Autodesk Inventor part; units mm, degrees
ref_plane "YZ Plane" through (0, 0, 0) normal (1, 0, 0) x (0, 1, 0)
ref_plane "XZ Plane" through (0, 0, 0) normal (0, 1, 0) x (-1, 0, 0)
ref_plane "XY Plane" through (0, 0, 0) normal (0, 0, 1) x (1, 0, 0)
sketch "Sketch1" plane through (0, 0, 0) normal (0, 0, 1) x (1, 0, 0)
  line L0 (-276.4159, 0) -> (46.0693, 0) construction
  line L1 (-22.2362, 22.2362) -> (0, 22.2362) construction
  line L2 (0, 22.2362) -> (0, 0)
  line L3 (0, 0) -> (-22.2362, 0)
  line L4 (-22.2362, 0) -> (-22.2362, 22.2362) construction
  line L5 (-22.2362, 22.2362) -> (0, 0) construction
  line L6 (0, 22.2362) -> (-22.2362, 0) construction
  line L7 (-230.3465, 421.1181) -> (-208.1103, 421.1181)
  line L8 (-208.1103, 421.1181) -> (-208.1103, 398.8819) construction
  line L9 (-208.1103, 398.8819) -> (-230.3465, 398.8819) construction
  line L10 (-230.3465, 398.8819) -> (-230.3465, 421.1181)
  line L11 (-230.3465, 421.1181) -> (-208.1103, 398.8819) construction
  line L12 (-208.1103, 421.1181) -> (-230.3465, 398.8819) construction
  line L13 (-230.3465, 398.8819) -> (-22.2362, 0)
  line L14 (-208.1103, 421.1181) -> (0, 22.2362)
  point P0 (-11.1181, 11.1181)
  point P1 (-219.2284, 410)
  dimension "d16" = 480
  dimension "d17" = 30
  dimension "d18" = 410
extrude "Extrusion1" add sketch "Sketch1" along normal mid plane 10
properties part number "Support - Left"
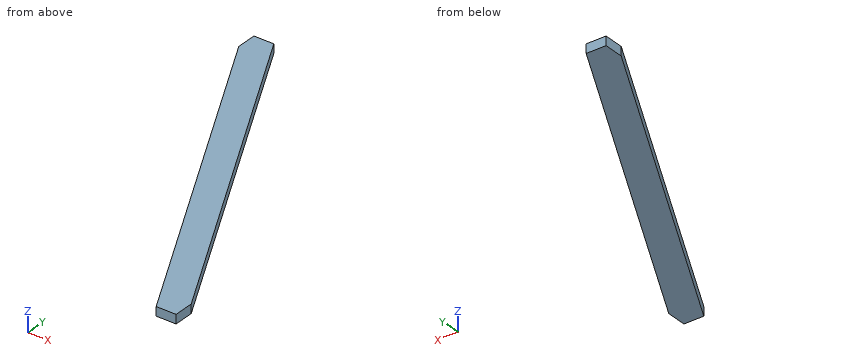
Work out the finished part from the listing and answer in its coordinate system (mm). Give positions to 0.01 mm unless a question says otherwise; leave off trailing zeros. Loops run counter-clockwise (first coordinate to the right, second up) from the corner with the lowest first, then second, coordinate; pieces in that order, holes last. Notation, with made-up numbers: (26, -13.5) -> (48, -13.5) arc R27 cw to (48, 9.5) -> close; hole circle Ø10 at (77.25, -1.75). An arc over 180 degrees is marked (long way). Use a Markdown table: item, result. Add a question column.
1) The part is cut by section C-C, the plane x = -129. Determine the outline of the cut face in (y, z).
2) Consider line 1 along X through (y, z) = (263, 1.25); line 2 along X through (y, z) = (335, 1.5); line 3 along Y through (x, z) = (-157.5, -3). Determine where each line is inside the solid, lowest interval first.
3) The part is cut by section A-A, the plane z = -1.5. Determine the outline of the cut face in (x, y), plus the area to 3 significant figures.
4) The part is cut by section B-B, the plane y = 251. Determine the outline of the cut face in (x, z), plus the area to 3 significant figures.
5) Each of these flat-tipped pins is pushed along its axis until it touches: P1, Ø4, axis at x = -26, z = -3.5, coming from the -Y side; P2, Ø6, axis at x = -196.5, z = -0.5, coming from the +Y side; P3, Ø3, axis at y = 349.5, z = -1.5, coming from the -X side. Where does it stop, or does it pass through?
Reported:
| question | item | result |
|---|---|---|
| 1 | outline | (204.63, -5) -> (269.49, -5) -> (269.49, 5) -> (204.63, 5) -> close |
| 2 | line 1 | x = -159.45 to -125.61 |
| 2 | line 2 | x = -197.02 to -163.18 |
| 2 | line 3 | y = 259.26 to 324.11 |
| 3 | outline | (-230.35, 398.88) -> (-22.24, 0) -> (0, 0) -> (0, 22.24) -> (-208.11, 421.12) -> (-230.35, 421.12) -> close |
| 3 | area | 14,000 mm^2 |
| 4 | outline | (-153.19, -5) -> (-119.35, -5) -> (-119.35, 5) -> (-153.19, 5) -> close |
| 4 | area | 338 mm^2 |
| 5 | P1 | stops at y = 3.38 |
| 5 | P2 | stops at y = 404.61 |
| 5 | P3 | stops at x = -205.36 |
